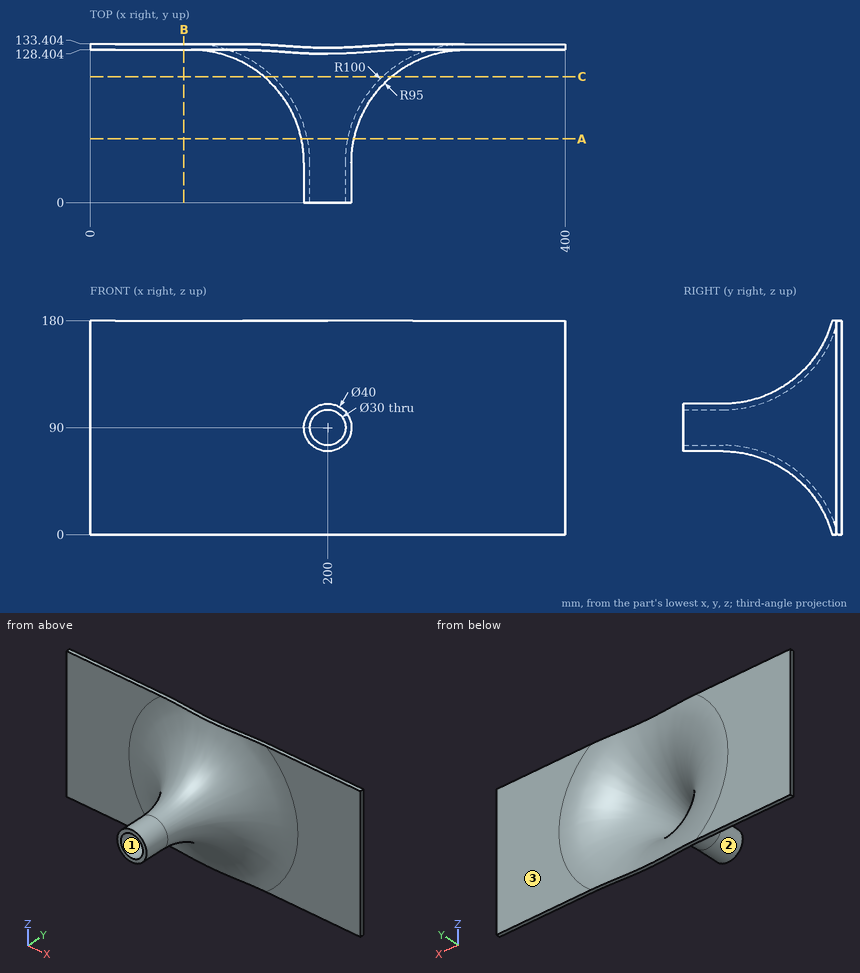
Here's the drawing with two shaded views (mm, measured from the low corner). I have some questions. Give positions to 0.01 mm unless a question says otherwise; leave off trailing zeros. Loops run counter-clockwise (first coordinate to the right, second up) from the corner with the lowest first, then second, coordinate; pieces in that order, holes last. Notation, with made-up numbers: (14, 0) - (72, 0) arc R20 cw to (72, 33) - close; hole circle Ø9 at (61, -11.5). An arc over 180 degrees is marked (long way). Answer in a Markdown table with one row per item. Add a question column.
Q1. Please list where these lines run through material, in increasing order: L1, parallel to X at y = 16, z = 90; L2, parallel to Y at x = 358.5, z = 154; L3, parallel to X at y = 13, z = 95.5 (1 decimal). Write a range as from..to.
Q2. We'd pull the mould along X, two halves only. Please class the marked faces 1, 2 and 3: +X half, -X half, draft (parallel to the pull), parting line (faces both ways), or undercut.
Q3. For pin 1 (5 mm diameter, centred on y = 96, z = 52.5, fed in from -X) (1 decimal); pin 2 (5 mm diameter, centred on x = 197, y = 83.5, fed in from -Z) (1 decimal); pin 3 (6 mm diameter, centred on y = 100.5, z = 125, fed in from +X) (1 decimal), each with a flat end and sliding along its axis, tell me the tip position at first contact or that it passes through.
Q4. If we section it at C-C (y = 106): List the corners of the cut face in (x, z) for me, plus the area to 3 significant figures.
Q5. If we section it at B-B (x = 79): List the corners of the cut face in (y, z) for me.
Q6. If we section it at A-A (y = 53.5): List the corners of the cut face in (x, z) for me.
The answers:
| question | item | result |
|---|---|---|
| 1 | L1 | x = 180..185, 215..220 |
| 1 | L2 | y = 128.4..133.4 |
| 1 | L3 | x = 180.8..186, 214..219.2 |
| 2 | face 1 | undercut |
| 2 | face 2 | parting line |
| 2 | face 3 | draft |
| 3 | pin 1 | stops at x = 172.4 |
| 3 | pin 2 | stops at z = 54.2 |
| 3 | pin 3 | stops at x = 237.7 |
| 4 | outline | circle Ø107.45 at (200, 90); hole circle Ø92.45 at (200, 90) |
| 4 | area | 2,350 mm^2 |
| 5 | outline | (128.4, 0) - (133.4, 0) - (133.4, 180) - (128.4, 180) - close |
| 6 | outline | circle Ø44.3 at (200, 90); hole circle Ø34.08 at (200, 90) |
